Here's how the part is built. I have some questions about the finished solid (model axes, mm). A direction names the side the tool comes from. Round coordinates to 2 decimals unless told otherwise and drop trailing zeros. Loops run counter-clockwise (first coordinate to the right, second up) from the corner with the lowest first, then second, coordinate; pieces in that order, holes last. Notation, with made-up numbers: M -40,-37.75 L 15,-37.75 A13 cw 15,-23.75 Z; hole C -5,-31.75 d11. An arc over 180 degrees is marked long. Put each result on its own line as item: value. Start each with the question number.
Autodesk Inventor part; units mm, degrees
ref_plane "YZ Plane" through (0, 0, 0) normal (1, 0, 0) x (0, 1, 0)
ref_plane "XZ Plane" through (0, 0, 0) normal (0, 1, 0) x (-1, 0, 0)
ref_plane "XY Plane" through (0, 0, 0) normal (0, 0, 1) x (1, 0, 0)
sketch "Sketch1" plane through (0, 0, 0) normal (0, 1, 0) x (-1, 0, 0)
  line L0 (0, 0) -> (26.25, 0)
  line L1 (26.25, 0) -> (26.25, -22)
  line L2 (26.25, -22) -> (0, -22)
  line L3 (0, -22) -> (0, 0)
  circle A0 centre (2, -20) radius 0.95
  circle A1 centre (24.25, -2) radius 1
  dimension "d0" = 26.25
  dimension "d1" = 22
  dimension "d3" = 1.9
  dimension "d6" = 2
  dimension "d18" = 2
  dimension "d19" = 2
  dimension "d20" = 2
  dimension "d21" = 2
extrude "Extrusion1" add sketch "Sketch1" along normal blind 1.1
sketch "Sketch2" plane through (0, 1.1, 0) normal (0, 1, 0) x (1, 0, 0)
  line L0 (0, 22) -> (-26.25, 22)
  line L1 (0, 0) -> (0, 22)
  line L2 (-22.625, 2.5) -> (-3.625, 2.5)
  line L3 (-3.625, 2.5) -> (-3.625, 19.5)
  line L4 (-3.625, 19.5) -> (-22.625, 19.5)
  line L5 (-22.625, 19.5) -> (-22.625, 2.5)
  line L6 (-22.625, 2.5) -> (-3.625, 19.5) construction
  line L7 (-3.625, 2.5) -> (-22.625, 19.5) construction
  point P0 (-13.125, 22)
  point P1 (0, 11)
  point P2 (-13.125, 11)
  point P3 (0, 11)
  point P4 (-13.125, 11)
  point P5 (-13.125, 22)
  point P6 (-13.125, 11)
  dimension "d11" = 19
  dimension "d12" = 17
extrude "Extrusion2" add sketch "Sketch2" along normal blind 11.3
sketch "Sketch3" plane through (0, 12.4, 0) normal (0, 1, 0) x (1, 0, 0)
  line L0 (-3.625, 2.5) -> (-3.625, 19.5) construction
  line L1 (-3.625, 19.5) -> (-22.625, 19.5) construction
  line L2 (-22.625, 19.5) -> (-22.625, 2.5) construction
  line L3 (-22.625, 2.5) -> (-3.625, 2.5) construction
  line L4 (-3.625, 19.5) -> (-3.625, 2.5) construction
  circle A0 centre (-13.125, 11) radius 7.5
  point P0 (0, 0)
  point P1 (-13.125, 19.5)
  point P2 (-3.625, 11)
  dimension "d15" = 15
extrude "Extrusion3" add sketch "Sketch3" along normal blind 15
sketch "Sketch4" plane through (0, 0, 0) normal (0, -1, 0) x (1, 0, 0)
  line L0 (-7.2, 0) -> (-12.7, 0)
  line L1 (-12.7, 0) -> (-12.7, -3.3)
  line L2 (-12.7, -3.3) -> (-7.2, -3.3)
  line L3 (-7.2, -3.3) -> (-7.2, 0)
  line L4 (0, 0) -> (-26.25, 0)
  circle A0 centre (-2, -20) radius 0.95
  dimension "d22" = 5.5
  dimension "d23" = 3.3
  dimension "d28" = 5.2
extrude "Extrusion4" add sketch "Sketch4" along normal blind 4.2 contours L3 L2 L1 L0
sketch "Sketch5" plane through (0, 0, 0) normal (0, -1, 0) x (1, 0, 0)
  line L0 (-4.3784, -18.3892) -> (-23.7162, -18.3892)
  line L1 (-23.7162, -18.3892) -> (-23.7162, -7.4432)
  line L2 (-23.7162, -7.4432) -> (-4.3784, -7.4432)
  line L3 (-4.3784, -7.4432) -> (-4.3784, -18.3892)
  point P0 (0, 0)
extrude "Extrusion5" add sketch "Sketch5" along normal blind 1.5
properties part number "camera_prz"
1) If we mould it in two halves opening along X, with no side actions, what happens to faces 1 (the face through (-25.174, 0.542, -1.617)), 2 (the face through (-3.625, 7, -11)), 3 (the face through (-13, 27.4, -11))? For each: pulls with the +X half, pulls with the -X half, needs draft (parallel to the pull), parting line crosses it, or undercut.
2) Suppose I cut it at C-C (z = -11). Write out the boundary of the cut face in (x, y) (3 decimals), plus the area to 3 significant figures.
3) On a 3-axis mill with a long thin cutter (end or side, diameter ignored), from which of +Z, -Z, +X, -X, +Y, -Y can I reach the whole of each face in a straight line? I mean faces 4 (the face through (-4.378, -1, -13)), 5 (the face through (-14, -1, -7.443)), 6 (the face through (-14.75, 19.79, -18.32)), 7 (the face through (-23.716, -1, -13)). Say none if no direction works.
4) If I drill on probe 1 along Z at (x, y) = (-2, 0.95); probe 2 along Z at (x, y) = (-24.25, 0.75); probe 3 along Z at (x, y) = (-17.5, 6), over which ranges is the centre line in solid material (lowest first)? Write a range as from..to.
5) Suppose I cut it at D-D (x = -22.25). Write out the boundary of the cut face in (y, z).
6) Suppose I cut it at A-A (z = -2). Write out the boundary of the cut face in (x, y).
7) I'm going to push flat-ended pins straight in: P1, Ø3.5, axis at x = -10.5, y = 9, coming from the -Z side; P2, Ø1.2, axis at x = -14, y = -1, coming from the +Z side; P3, Ø10, axis at x = -21.5, z = -7, coming from the -Y side; P4, Ø12, axis at y = -0.5, z = -6, coming from the -X side. Where does each tip first touch, or does it pass through?
8) Suppose I cut it at B-B (x = -2). Write out the boundary of the cut face in (y, z).
Results are:
1. face 1: undercut
1. face 2: pulls with the +X half
1. face 3: needs draft
2. outline: M -26.25,0 L -23.716,0 L -23.716,-1.5 L -4.378,-1.5 L -4.378,0 L 0,0 L 0,1.1 L -3.625,1.1 L -3.625,12.4 L -5.625,12.4 L -5.625,27.4 L -20.625,27.4 L -20.625,12.4 L -22.625,12.4 L -22.625,1.1 L -26.25,1.1 Z
2. area: 498 mm²
3. face 4: +Z, -Z, +X, -Y
3. face 5: +X, -X, -Y
3. face 6: +Y
3. face 7: +Z, -Z, -X, -Y
4. probe 1: -22..-20.95, -19.05..0
4. probe 2: -22..-3, -1..0
4. probe 3: -19.5..-2.5
5. outline: M -1.5,-18.39 L 0,-18.39 L 0,-22 L 1.1,-22 L 1.1,-19.5 L 12.4,-19.5 L 12.4,-2.5 L 1.1,-2.5 L 1.1,0 L 0,0 L 0,-7.44 L -1.5,-7.44 Z
6. outline: M -26.25,0 L -25.25,0 L -25.25,1.1 L -26.25,1.1 Z; M -23.25,0 L -12.7,0 L -12.7,-4.2 L -7.2,-4.2 L -7.2,0 L 0,0 L 0,1.1 L -23.25,1.1 Z
7. P1: z = -19.5
7. P2: z = -7.44
7. P3: y = -1.5
7. P4: x = -26.25
8. outline: M 0,-22 L 1.1,-22 L 1.1,-20.95 L 0,-20.95 Z; M 0,-19.05 L 1.1,-19.05 L 1.1,0 L 0,0 Z
